Check sheet for the modelled part. Datum: model origin and axes. Units: mm. Face numbers are marked on the shaded views. A direction names the side the tool comes from. Round coordinates to 2 decimals unless told otherwise and drop trailing zeros. Loops run counter-clockwise (first coordinate to the right, second up) from the corner with the lowest first, then second, coordinate; pieces in that order, holes last. Notation, with made-up numbers: (-36, -15) - (-8, -15) arc R20 ccw to (-8, 19) - close; hole circle Ø6 at (-36.5, 30.5). An arc over 180 degrees is marked (long way). Return JSON: item names as keys, results as strings.
from build123d import *

# Parameters (mm, degrees)
SKETCH1_R           = 6.2738
SKETCH1_R_2         = 3.175
BOSS_EXTRUDE1_DEPTH = 22.86
SKETCH2_W           = 25.4
SKETCH2_H           = 22.86
BOSS_EXTRUDE2_DEPTH = 1.27
FILLET1_R           = 2.54
SKETCH3_R           = 6.2738
CUT_EXTRUDE1_DEPTH  = 16.51
CUT_EXTRUDE5_START  = 3.175
CUT_EXTRUDE5_DEPTH  = 10.16
BOSS_EXTRUDE4_DEPTH = 22.86
FILLET2_R           = 2.54
FILLET3_R           = 2.54
BOSS_EXTRUDE5_DEPTH = 22.86


with BuildPart() as part:
    # Sketch1 → Boss-Extrude1 (new body)
    with BuildSketch(Plane.XY):
        Circle(SKETCH1_R)
        Circle(SKETCH1_R_2, mode=Mode.SUBTRACT)
    boss_extrude1 = extrude(amount=BOSS_EXTRUDE1_DEPTH)

    # Sketch2 → Boss-Extrude2 (add)
    with BuildSketch(Plane(origin=(0, 6.2738, 0), x_dir=(1, 0, 0), z_dir=(0, 1, 0))):
        with Locations((12.7, -11.43)):
            Rectangle(SKETCH2_W, SKETCH2_H)
    boss_extrude2 = extrude(amount=-BOSS_EXTRUDE2_DEPTH)

    # Fillet1
    fillet1_edges = [part.edges().sort_by_distance(p)[0] for p in [
        (3.784514764, 5.0038, 11.43),
    ]]
    fillet(fillet1_edges, radius=FILLET1_R)

    # Sketch3 → Cut-Extrude1 (cut)
    with BuildSketch(Plane(origin=(0, 0, 3.175), x_dir=(-1, 0, 0), z_dir=(0, 0, -1))):
        Circle(SKETCH3_R)
    cut_extrude1 = extrude(amount=-CUT_EXTRUDE1_DEPTH, mode=Mode.SUBTRACT)

    # Sketch9 → Cut-Extrude5 (cut)
    with BuildSketch(Plane(origin=(0, 0, 19.685), x_dir=(-1, 0, 0), z_dir=(0, 0, -1)).offset(CUT_EXTRUDE5_START)):
        with BuildLine():
            Line((-6.2738, 0), (-8.462432274, 5.0038))
            Line((-8.462432274, 5.0038), (-3.784514764, 5.0038))
            ThreePointArc((-3.784514764, 5.0038), (5.617110252, -2.794394184), (-6.2738, 0))
        make_face()
    extrude(amount=CUT_EXTRUDE5_DEPTH, mode=Mode.SUBTRACT)

    # Sketch10 → Boss-Extrude4 (add)
    with BuildSketch(Plane.XY.offset(22.86)):
        with BuildLine():
            Line((0, 6.2738), (0, 19.05))
            Line((0, 19.05), (4.7625, 19.05))
            Line((4.7625, 19.05), (4.7625, 4.084012756))
            ThreePointArc((4.7625, 4.084012756), (2.620905112, 5.700124809), (0, 6.2738))
        make_face()
    boss_extrude4 = extrude(amount=-BOSS_EXTRUDE4_DEPTH)

    # Fillet2
    fillet2_edges = [part.edges().sort_by_distance(p)[0] for p in [
        (4.7625, 6.2738, 11.43),
    ]]
    fillet(fillet2_edges, radius=FILLET2_R)

    # Mirror5: Boss-Extrude4 across plane
    add(boss_extrude4.mirror(Plane(origin=(4.7625, 19.05, -15.705482496), x_dir=(0, 0, 1), z_dir=(0, 1, 0))))

    # Mirror7: Boss-Extrude1 across plane
    add(boss_extrude1.mirror(Plane.ZX.offset(18.9738)))

    # Mirror9: Boss-Extrude2 across plane
    add(boss_extrude2.mirror(Plane.ZX.offset(18.9738)))

    # Mirror11: Cut-Extrude1 across plane
    add(cut_extrude1.mirror(Plane.ZX.offset(18.9738)), mode=Mode.SUBTRACT)

    # Fillet3
    fillet3_edges = [part.edges().sort_by_distance(p)[0] for p in [
        (4.7625, 31.6738, 11.43),
    ]]
    fillet(fillet3_edges, radius=FILLET3_R)

    # Sketch12 → Boss-Extrude5 (add)
    with BuildSketch(Plane.XY.offset(22.86)):
        with BuildLine():
            Line((8.462432274, 32.9438), (4.7625, 32.9438))
            Line((4.7625, 32.9438), (4.7625, 36.451836926))
            Line((4.7625, 36.451836926), (6.023690985, 36.193828818))
            ThreePointArc((6.023690985, 36.193828818), (6.430798302, 33.959312086), (8.462432274, 32.9438))
        make_face()
    extrude(amount=-BOSS_EXTRUDE5_DEPTH)


solid = part.part
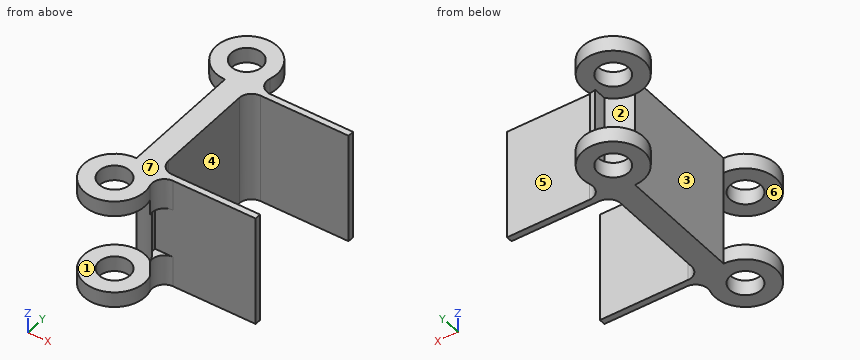
Q1. Sectioned sample at B-B (x = 13). Enter the section's corners in (y, z).
Answer key:
{"outline": "(5, 0) - (6.27, 0) - (6.27, 22.86) - (5, 22.86) - close; (31.67, 0) - (32.94, 0) - (32.94, 22.86) - (31.67, 22.86) - close"}
Q2. Tool access check on the marked faces 1, 2, 3 and 4. Record the directions out of +Z, -Z, +X, -X, +Y, -Y that give a thin tool (end or side, any length) a straight path to the whole face; none if there is none.
Answer key:
{"face 1": "-X, -Y", "face 2": "-X, +Y", "face 3": "+Z, -Z, -X", "face 4": "+Z, -Z, +X"}
Q3. Scan lines: probe 1 along Y at (x, z) = (23.5, 7.75); probe 2 along Y at (x, z) = (-1.5, 2.5); probe 3 along X at (y, z) = (22, 9.5). Record each from-to range of solid material in increasing order. Write a range as [from, to].
Answer key:
{"probe 1": "y = [5, 6.27], [31.67, 32.94]", "probe 2": "y = [-6.09, -2.8], [2.8, 6.09], [31.86, 35.15], [40.75, 44.04]", "probe 3": "x = [0, 4.76]"}
Q4. Sectioned sample at D-D (z = 20.25). State how many separate pieces and enclosed holes the cut face has, plus the area to 3 significant figures.
Answer key:
{"separate pieces": "1", "enclosed holes": "2", "area": "373 mm²"}
Q5. Sectioned sample at A-A (y = 0). Enter the section's corners in (x, z) (3 decimals), plus the area to 3 significant figures.
Answer key:
{"outline": "(-6.274, 0) - (-3.175, 0) - (-3.175, 3.175) - (-6.274, 3.175) - close; (-6.274, 19.685) - (-3.175, 19.685) - (-3.175, 22.86) - (-6.274, 22.86) - close; (3.175, 0) - (6.274, 0) - (6.274, 3.175) - (3.175, 3.175) - close; (3.175, 19.685) - (6.274, 19.685) - (6.274, 22.86) - (3.175, 22.86) - close", "area": "39.4 mm²"}
Q6. Depth check by flat-ended pin: P1, Ø5, axis at x = 12, z = 6, coming from the +Y side; P2, Ø12, axis at y = 28, z = 19, coming from the -X side; P3, Ø3, axis at y = 12.5, z = 16, coming from the +X side. Enter the tip coordinate at first touch or a pass-through.
Answer key:
{"P1": "stops at y = 32.94", "P2": "stops at x = -4.84", "P3": "stops at x = 4.76"}
Q7. Draft check along Z on the marked faces 5, 6 and 7. Enter one of: released by +Z, released by -Z, zero draft, split by the parting line, or undercut.
Answer key:
{"face 5": "zero draft", "face 6": "undercut", "face 7": "released by +Z"}
Q8. Sectioned sample at C-C (z = 5.5). Enter the section's corners in (x, y).
Answer key:
{"outline": "(0, 6.27) arc R6.27 cw to (6.02, 1.75) arc R2.54 cw to (8.46, 5) - (25.4, 5) - (25.4, 6.27) - (7.3, 6.27) arc R2.54 cw to (4.76, 8.81) - (4.76, 29.13) arc R2.54 cw to (7.3, 31.67) - (25.4, 31.67) - (25.4, 32.94) - (8.46, 32.94) arc R2.54 cw to (6.02, 36.19) - (4.76, 36.45) - (4.76, 33.86) arc R6.27 cw to (0, 31.67) - close"}
